Design review of the part shown in the three views and the two pictorial views. Dimensions are in mm from the part's minimum x, y and z. A direction names the side the tool comes from. Coordinates: 2 decimals unless noted, no trailing zeros. Write each loop counter-clockwise with the first axis right and the second up, starting at its lowest first coordinate (ties: lowest second). Pieces come first, ordered by that corner, then holes. Notation, with made-up numbers: (-31.75, 69.5) -> (-15.75, 69.5) arc R14 cw to (-15.75, 88.5) -> close; hole circle Ø4 at (-21, -32.75). An arc over 180 degrees is marked (long way). Write each question's results on one line, items separated by ' | '.
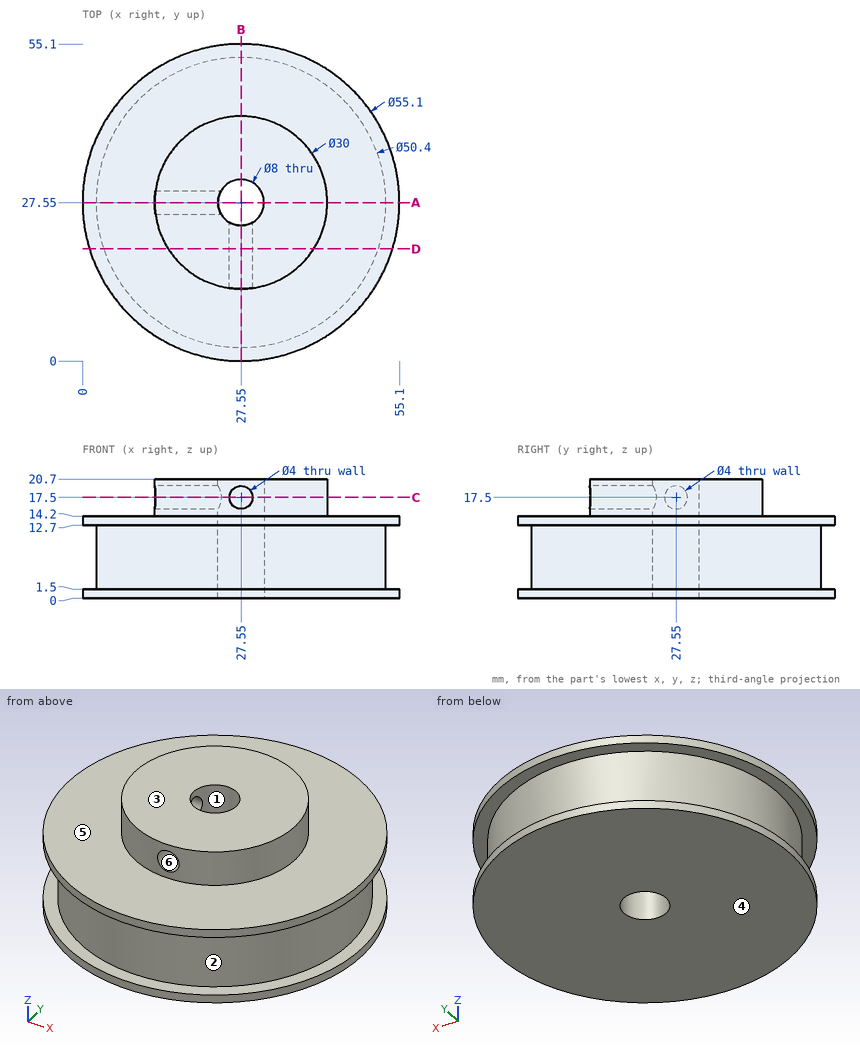
Q1. Machinability: for the marked faces 4, 5 and 6, which of the approach directions +Z, -Z, +X, -X, +Y, -Y give a long, thin tool a straight path to every point of the face, cutting with its end or side? Answer none if there is none.
Solution:
face 4: -Z, +X, -X, +Y, -Y | face 5: +Z | face 6: -Y
Q2. For line 1 (Z direction, x = 3, y = 16); line 2 (Y direction, x = 27.55, z = 12.25); line 3 (Z direction, x = 26, y = 42.5), list the stretches that pass through material, from the lowest coordinate up. Write a range as from..to.
Solution:
line 1: 0..1.5, 12.7..14.2 | line 2: 2.35..23.55, 31.55..52.75 | line 3: 0..14.2
Q3. Add section C-C (z = 17.5). Write out the cut boundary in (x, y).
Solution:
outline: (12.68, 25.55) arc R15 ccw to (25.55, 12.68) -> (25.55, 24.09) arc R4 cw to (24.09, 25.55) -> close; (12.68, 29.55) -> (24.09, 29.55) arc R4 cw (long way) to (29.55, 24.09) -> (29.55, 12.68) arc R15 ccw (long way) to start
Q4. Clearance check with flat-ended pins moving along their axes: P1, Ø2, axis at x = 38, z = 13, coming from the +Y side; P2, Ø3, axis at x = 27.55, z = 17.5, coming from the +Y side; P3, Ø5, axis at y = 16, z = 13.5, coming from the +X side; P4, Ø5, axis at x = 40.5, y = 39, coming from the +Z side. State where each tip first meets the part, or that it passes through.
Solution:
P1: y = 53.43 | P2: y = 42.55 | P3: x = 53.57 | P4: z = 20.7
Q5. Add section D-D (y = 19.5). Write out the cut boundary in (x, z).
Solution:
outline: (1.2, 0) -> (53.9, 0) -> (53.9, 1.5) -> (51.43, 1.5) -> (51.43, 12.7) -> (53.9, 12.7) -> (53.9, 14.2) -> (40.21, 14.2) -> (40.21, 20.7) -> (14.89, 20.7) -> (14.89, 14.2) -> (1.2, 14.2) -> (1.2, 12.7) -> (3.67, 12.7) -> (3.67, 1.5) -> (1.2, 1.5) -> close; hole circle Ø4 at (27.55, 17.5)
Q6. Add section A-A (y = 27.55). Write out the cut boundary in (x, z).
Solution:
outline: (0, 0) -> (23.55, 0) -> (23.55, 15.5) -> (12.55, 15.5) -> (12.55, 14.2) -> (0, 14.2) -> (0, 12.7) -> (2.35, 12.7) -> (2.35, 1.5) -> (0, 1.5) -> close; (12.55, 19.5) -> (23.55, 19.5) -> (23.55, 20.7) -> (12.55, 20.7) -> close; (31.55, 0) -> (55.1, 0) -> (55.1, 1.5) -> (52.75, 1.5) -> (52.75, 12.7) -> (55.1, 12.7) -> (55.1, 14.2) -> (42.55, 14.2) -> (42.55, 20.7) -> (31.55, 20.7) -> close
Q7. Draft analysis for pull direction X (two halves, no side actions). For the marked faces 1, 2 and 3, state which applies: pulls with the +X half, pulls with the -X half, needs draft (parallel to the pull), parting line crosses it, or undercut.
Solution:
face 1: undercut | face 2: parting line crosses it | face 3: needs draft
